The listing builds one solid part. Answer for the finished solid, in the listing's coordinates (mm). A direction names the side the tool comes from. Give positions to 0.01 mm unless a question says otherwise; leave off trailing zeros. Loops run counter-clockwise (first coordinate to the right, second up) from the corner with the lowest first, then second, coordinate; pieces in that order, holes last. Notation, with made-up numbers: M -33.5,-37 L 14.5,-37 A19 cw 14.5,-32 Z; hole C 58.25,-2 d8. An arc over 180 degrees is marked long. Return JSON: item names as keys, results as strings.
from build123d import *

# Parameters (mm, degrees)
SIDE_W         = 22.5
SIDE_H         = 7.5
SIDE_EX_DEPTH  = 6.5
HOLE_R         = 1.5
HOLE_CUT_DEPTH = 25.591665255
WIRE_CUT_DEPTH = 25.591665255
FILLET1_R      = 1


with BuildPart() as part:
    # Side → Side_Ex (new body)
    with BuildSketch(Plane(origin=(0, 0, 0), x_dir=(1, 0, 0), z_dir=(0, 1, 0))):
        with Locations((11.25, 3.75)):
            Rectangle(SIDE_W, SIDE_H)
    extrude(amount=SIDE_EX_DEPTH)

    # Hole → Hole_Cut (cut, through all)
    with BuildSketch(Plane(origin=(0, 0, -7.5), x_dir=(-1, 0, 0), z_dir=(0, 0, -1))):
        with Locations((-4, 3.25)):
            Circle(HOLE_R)
    extrude(amount=-HOLE_CUT_DEPTH, mode=Mode.SUBTRACT)

    # Wire 2 → Wire_Cut (cut, through all)
    with BuildSketch(Plane(origin=(0, 0, 0), x_dir=(1, 0, 0), z_dir=(0, 1, 0))):
        with BuildLine():
            Line((16.7, 5.5), (9.8, 5.5))
            ThreePointArc((9.8, 5.5), (8.527207794, 4.972792206), (8, 3.7))
            Line((8, 3.7), (8, 0))
            Line((8, 0), (18.5, 0))
            Line((18.5, 0), (18.5, 3.7))
            ThreePointArc((18.5, 3.7), (17.972792206, 4.972792206), (16.7, 5.5))
        make_face()
    extrude(amount=WIRE_CUT_DEPTH, mode=Mode.SUBTRACT)

    # Fillet1
    fillet1_edges = [part.edges().sort_by_distance(p)[0] for p in [
        (11.25, 6.5, -7.5),
        (11.25, 0, -7.5),
        (0, 3.25, -7.5),
        (22.5, 3.25, -7.5),
    ]]
    fillet(fillet1_edges, radius=FILLET1_R)


solid = part.part
(1) Determine the mould class of faces 1 (the cylindrical face through (8.541, 3.204, -4.987)), 2 (the cylindrical face through (0.285, 3.295, -7.199)), 3 (the flat face through (20, 3, 0)), 4 (the cylindrical face through (22.199, 3.295, -7.215)) for opening direction X: released by +X, released by -X, zero draft, split by the parting line, or undercut.
Values follow:
{"face 1": "undercut", "face 2": "released by -X", "face 3": "zero draft", "face 4": "released by +X"}
(2) The part is cut by section D-D (z = -4.75). Determine the outline of the cut face in (x, y).
Values follow:
{"outline": "M 0,0 L 8.34,0 L 8.34,6.5 L 0,6.5 Z; M 18.16,0 L 22.5,0 L 22.5,6.5 L 18.16,6.5 Z; hole C 4,3.25 d3"}
(3) The part is cut by section A-A (z = -2). Determine the outline of the cut face in (x, y).
Values follow:
{"outline": "M 0,0 L 8,0 L 8,6.5 L 0,6.5 Z; M 18.5,0 L 22.5,0 L 22.5,6.5 L 18.5,6.5 Z; hole C 4,3.25 d3"}
(4) The part is cut by section C-C (x = 4). Determine the outline of the cut face in (y, z), and give its area (3 significant figures).
Values follow:
{"outline": "M 0,-6.5 A1 ccw 1,-7.5 L 1.75,-7.5 L 1.75,0 L 0,0 Z; M 4.75,-7.5 L 5.5,-7.5 A1 ccw 6.5,-6.5 L 6.5,0 L 4.75,0 Z", "area": "25.8 mm²"}
(5) The part is cut by section B-B (y = 3.25). Determine the outline of the cut face in (x, z).
Values follow:
{"outline": "M 0,-6.5 A1 ccw 1,-7.5 L 2.5,-7.5 L 2.5,0 L 0,0 Z; M 5.5,-7.5 L 21.5,-7.5 A1 ccw 22.5,-6.5 L 22.5,0 L 18.5,0 L 18.5,-3.7 A1.8 cw 16.7,-5.5 L 9.8,-5.5 A1.8 cw 8,-3.7 L 8,0 L 5.5,0 Z"}
(6) Given pin 1 (2 mm diameter, centred on x = 14.5, y = 4.5, fed in from +Z); pin 2 (2.5 mm diameter, centred on x = 4, y = 3.25, fed in from +Z), each flat-ended and moving along its own axis, determine where each tip first touches the part or whether it passes through.
Values follow:
{"pin 1": "z = -5.5", "pin 2": "through"}
(7) A tool of negligible diameter and unlimited length cuts with its end or side. For faces 5 (the cylindrical face through (17.987, 3.204, -4.959)), 6 (the flat face through (4.8, 1.8, 0)), from which of +Z, -Z, +X, -X, +Y, -Y can it reach the whole face along a straight path? Write none if from no direction.
Values follow:
{"face 5": "+Z, +Y, -Y", "face 6": "+Z, +X, -X, +Y, -Y"}
(8) Straight lines are drawn through the part: line 1 along Y through (x, z) = (4, -5.75); line 2 along X through (y, z) = (2.5, -0.5); line 3 along X through (y, z) = (3.75, -4.75). For each, find the intervals that lie inside material, in ascending order.
Values follow:
{"line 1": "0 to 1.75, 4.75 to 6.5", "line 2": "0 to 2.7, 5.3 to 8, 18.5 to 22.5", "line 3": "0 to 2.59, 5.41 to 8.34, 18.16 to 22.5"}
